Design review of the part built by this model. Coordinates are the model's own, in mm. Coordinates: 2 decimals unless noted, no trailing zeros. Order: outer loops, then holes, each group sorted by start corner. A loop starts at its lowest first (then second) coordinate and runs counter-clockwise, first axis right, second up. Notation, with made-up numbers: (27, 87) -> (43, 87) arc R27 cw to (43, 104) -> close; hole circle Ø8 at (-1, 31). An arc over 180 degrees is marked (long way). Use a Markdown table: item, result. Add a question column.
Q1. Add section B-B (y = -10). State the section outline as (x, z) points.
Q2. Add section A-A (x = 40). State the section outline as (y, z) points.
Q3. Wall thickness on probe 1 along Y at (x, z) = (40, 2.45); probe 2 along Y at (x, z) = (-37.1, 2.35); probe 3 along Y at (x, z) = (-20, 0.8): over which ranges is each line inside the solid? List them lowest first.
Q4. Add section D-D (x = -20). State the section outline as (y, z) points.
Q5. Add section C-C (y = 38). State the section outline as (x, z) points.
Q6. The part is to be moulded in two halves that separate along Y. For faces 1 (the face through (-50, -1, 1)), 2 (the face through (-34.79, -0.96, 1.52)), 3 (the face through (1, -44, 1)), 4 (the face through (-48.98, 43.04, 1.52)), say which applies: pulls with the +Y half, pulls with the -Y half, needs draft (parallel to the pull), parting line crosses it, or undercut.
Autodesk Inventor part; units mm, degrees
ref_plane "YZ Plane" through (0, 0, 0) normal (1, 0, 0) x (0, 1, 0)
ref_plane "XZ Plane" through (0, 0, 0) normal (0, 1, 0) x (-1, 0, 0)
ref_plane "XY Plane" through (0, 0, 0) normal (0, 0, 1) x (1, 0, 0)
sketch "Sketch1" plane through (0, 0, 0) normal (0, 0, 1) x (1, 0, 0)
  line L0 (-50, 44) -> (50, 44)
  line L1 (50, 44) -> (50, -44)
  line L2 (50, -44) -> (-50, -44)
  line L3 (-50, -44) -> (-50, 44)
  line L4 (0, 44) -> (0, -44) construction
  line L5 (-50, 0) -> (50, 0) construction
  point P0 (0, 0)
  dimension "d0" = 100
  dimension "d1" = 88
extrude "Extrusion1" add sketch "Sketch1" along normal blind 3
sketch "Sketch2" plane through (0, 0, 3) normal (0, 0, 1) x (1, 0, 0)
  line L0 (-50, 44) -> (-50, -44)
  line L1 (50, -44) -> (50, 44)
  circle A0 centre (0, 0) radius 2.5
  circle A1 centre (0, 10) radius 2.5
  line L2 (0, 0) -> (0, 20.5611) construction
  circle A2 centre (-10, 0) radius 2.5
  circle A3 centre (0, -10) radius 2.5
  circle A4 centre (10, 0) radius 2.5
  circle A5 centre (-37.1, 0) radius 2.5
  circle A6 centre (-37.1, -10) radius 2.5
  circle A7 centre (-37.1, -20) radius 2.5
  circle A8 centre (-37.1, 10) radius 2.5
  circle A9 centre (-37.1, 0) radius 2.5
  circle A10 centre (-37.1, -10) radius 2.5
  circle A11 centre (-37.1, 20) radius 2.5
  circle A12 centre (-37.1, 10) radius 2.5
  circle A13 centre (-37.1, 0) radius 2.5
  line L3 (0, 0) -> (-50, 0) construction
  circle A14 centre (40, 0) radius 3.6 construction
  circle A15 centre (40, 20) radius 3.6 construction
  circle A16 centre (40, -20) radius 3.6 construction
  circle A17 centre (40, 0) radius 3.6 construction
  circle A18 centre (40, 0) radius 3.6
  line L4 (40, 0) -> (40, 20) construction
  line L5 (40, 0) -> (40, -20) construction
  circle A19 centre (40, 20) radius 2.5
  circle A20 centre (40, -20) radius 2.5
  dimension "d40" = 6.5
  dimension "d4" = 5
  dimension "d5" = 5
  dimension "d6" = 10
  dimension "d9" = 360
  dimension "d11" = 5
  dimension "d12" = 12.9
  dimension "d15" = 10
  dimension "d18" = 10
  dimension "d28" = 20
  dimension "d31" = 20
  dimension "d64" = 7.2
  dimension "d65" = 5
  dimension "d66" = 5
extrude "Extrusion2" cut sketch "Sketch2" against normal up to next
sketch "Sketch3" plane through (0, 0, 3) normal (0, 0, 1) x (1, 0, 0)
  circle A0 centre (0, 0) radius 2.5
  line L0 (50, 44) -> (-50, 44)
  line L1 (-50, -44) -> (50, -44)
  line L2 (0, 0) -> (0, -39.6664) construction
  line L3 (0, 0) -> (-44.4767, 0) construction
  line L4 (-3.25, -38) -> (3.25, -38) construction
  line L5 (-3.25, -39.5) -> (3.25, -39.5)
  line L6 (3.25, -36.5) -> (-3.25, -36.5)
  arc A1 (-3.25, -36.5) -> (-3.25, -39.5) centre (-3.25, -38) ccw
  arc A2 (3.25, -39.5) -> (3.25, -36.5) centre (3.25, -38) ccw
  line L7 (16.9, -38) -> (23.4, -38) construction
  line L8 (16.9, -39.5) -> (23.4, -39.5)
  line L9 (23.4, -36.5) -> (16.9, -36.5)
  arc A3 (16.9, -36.5) -> (16.9, -39.5) centre (16.9, -38) ccw
  arc A4 (23.4, -39.5) -> (23.4, -36.5) centre (23.4, -38) ccw
  line L10 (-23.4, -38) -> (-16.9, -38) construction
  line L11 (-23.4, -39.5) -> (-16.9, -39.5)
  line L12 (-16.9, -36.5) -> (-23.4, -36.5)
  arc A5 (-23.4, -36.5) -> (-23.4, -39.5) centre (-23.4, -38) ccw
  arc A6 (-16.9, -39.5) -> (-16.9, -36.5) centre (-16.9, -38) ccw
  line L13 (-3.25, -38) -> (3.25, -38) construction
  line L14 (-3.25, -39.5) -> (3.25, -39.5)
  line L15 (3.25, -36.5) -> (-3.25, -36.5)
  arc A7 (-3.25, -36.5) -> (-3.25, -39.5) centre (-3.25, -38) ccw
  arc A8 (3.25, -39.5) -> (3.25, -36.5) centre (3.25, -38) ccw
  line L16 (-3.25, 38) -> (3.25, 38) construction
  line L17 (-3.25, 39.5) -> (3.25, 39.5)
  line L18 (3.25, 36.5) -> (-3.25, 36.5)
  arc A9 (-3.25, 39.5) -> (-3.25, 36.5) centre (-3.25, 38) ccw
  arc A10 (3.25, 36.5) -> (3.25, 39.5) centre (3.25, 38) ccw
  arc A11 (16.9, 39.5) -> (16.9, 36.5) centre (16.9, 38) ccw
  line L19 (23.4, 36.5) -> (16.9, 36.5)
  line L20 (16.9, 38) -> (23.4, 38) construction
  line L21 (16.9, 39.5) -> (23.4, 39.5)
  arc A12 (23.4, 36.5) -> (23.4, 39.5) centre (23.4, 38) ccw
  arc A13 (-23.4, 39.5) -> (-23.4, 36.5) centre (-23.4, 38) ccw
  line L22 (-16.9, 36.5) -> (-23.4, 36.5)
  line L23 (-23.4, 38) -> (-16.9, 38) construction
  line L24 (-23.4, 39.5) -> (-16.9, 39.5)
  arc A14 (-16.9, 36.5) -> (-16.9, 39.5) centre (-16.9, 38) ccw
  arc A15 (-3.25, 39.5) -> (-3.25, 36.5) centre (-3.25, 38) ccw
  line L25 (3.25, 36.5) -> (-3.25, 36.5)
  line L26 (-3.25, 38) -> (3.25, 38) construction
  line L27 (-3.25, 39.5) -> (3.25, 39.5)
  arc A16 (3.25, 36.5) -> (3.25, 39.5) centre (3.25, 38) ccw
  line L28 (50, -44) -> (-50, -44)
  line L29 (0, -44) -> (0, -31) construction
  line L30 (-10.32, -31) -> (10.32, -31) construction
  line L31 (-10.32, -33.5) -> (10.32, -33.5)
  line L32 (10.32, -28.5) -> (-10.32, -28.5)
  arc A17 (-10.32, -28.5) -> (-10.32, -33.5) centre (-10.32, -31) ccw
  arc A18 (10.32, -33.5) -> (10.32, -28.5) centre (10.32, -31) ccw
  line L33 (-10.32, 33.5) -> (10.32, 33.5)
  line L34 (10.32, 28.5) -> (-10.32, 28.5)
  arc A19 (-10.32, 33.5) -> (-10.32, 28.5) centre (-10.32, 31) ccw
  line L35 (0, 44) -> (0, 31) construction
  line L36 (-10.32, 31) -> (10.32, 31) construction
  line L37 (-10.32, 33.5) -> (10.32, 33.5)
  line L38 (10.32, 28.5) -> (-10.32, 28.5)
  arc A20 (-10.32, 33.5) -> (-10.32, 28.5) centre (-10.32, 31) ccw
  arc A21 (10.32, 28.5) -> (10.32, 33.5) centre (10.32, 31) ccw
  point P0 (0, -38)
  point P1 (20.15, -38)
  point P2 (-20.15, -38)
  point P3 (0, -38)
  point P4 (0, 38)
  point P5 (20.15, 38)
  point P6 (-20.15, 38)
  point P7 (0, 38)
  dimension "d38" = 3
  dimension "d40" = 6.5
  dimension "d43" = 20.15
  dimension "d46" = 20.15
  dimension "d59" = 6
  dimension "d61" = 13
  dimension "d62" = 10.32
  dimension "d63" = 5
extrude "Extrusion3" cut sketch "Sketch3" against normal up to next contours A1 L6 A2 L5 | A3 L9 A4 L8 | A5 L12 A6 L11 | L17 A10 L18 A9 | L21 A12 L19 A11 | L24 A14 L22 A13 | A17 L32 A18 L31 | L33 A21 L34 A19
fillet "Fillet1" radius 3.38 4 edges at (50, -44, 1.5) (50, 44, 1.5) (-50, -44, 1.5) (-50, 44, 1.5)
sketch "Sketch5" plane through (0, 0, 3) normal (0, 0, 1) x (1, 0, 0)
  line L0 (-20, 20) -> (20, 20) construction
  line L1 (20, 20) -> (20, -20) construction
  line L2 (20, -20) -> (-20, -20) construction
  line L3 (-20, -20) -> (-20, 20) construction
  circle A0 centre (0, 0) radius 2.5
  line L4 (-20, 20) -> (20, -20) construction
  line L5 (20, 20) -> (-20, -20) construction
  circle A1 centre (-20, 20) radius 2.75
  circle A2 centre (20, 20) radius 2.75
  circle A3 centre (-20, -20) radius 2.75
  circle A4 centre (20, -20) radius 2.75
  dimension "d67" = 40
  dimension "d68" = 40
  dimension "d69" = 5.5
  dimension "d70" = 5.5
  dimension "d71" = 5.5
  dimension "d72" = 5.5
extrude "Extrusion5" cut sketch "Sketch5" against normal through all contours A1 | A2 | A3 | A4
properties part number "20mm gantry plate" material "Aluminum 6061"
Established:
| question | item | result |
|---|---|---|
| 1 | outline | (-50, 0) -> (-39.6, 0) -> (-39.6, 3) -> (-50, 3) -> close; (-34.6, 0) -> (-2.5, 0) -> (-2.5, 3) -> (-34.6, 3) -> close; (2.5, 0) -> (50, 0) -> (50, 3) -> (2.5, 3) -> close |
| 2 | outline | (-44, 0) -> (-22.5, 0) -> (-22.5, 3) -> (-44, 3) -> close; (-17.5, 0) -> (-3.6, 0) -> (-3.6, 3) -> (-17.5, 3) -> close; (3.6, 0) -> (17.5, 0) -> (17.5, 3) -> (3.6, 3) -> close; (22.5, 0) -> (44, 0) -> (44, 3) -> (22.5, 3) -> close |
| 3 | probe 1 | -44 to -22.5, -17.5 to -3.6, 3.6 to 17.5, 22.5 to 44 |
| 3 | probe 2 | -44 to -22.5, -17.5 to -12.5, -7.5 to -2.5, 2.5 to 7.5, 12.5 to 17.5, 22.5 to 44 |
| 3 | probe 3 | -44 to -39.5, -36.5 to -22.75, -17.25 to 17.25, 22.75 to 36.5, 39.5 to 44 |
| 4 | outline | (-44, 0) -> (-39.5, 0) -> (-39.5, 3) -> (-44, 3) -> close; (-36.5, 0) -> (-22.75, 0) -> (-22.75, 3) -> (-36.5, 3) -> close; (-17.25, 0) -> (17.25, 0) -> (17.25, 3) -> (-17.25, 3) -> close; (22.75, 0) -> (36.5, 0) -> (36.5, 3) -> (22.75, 3) -> close; (39.5, 0) -> (44, 0) -> (44, 3) -> (39.5, 3) -> close |
| 5 | outline | (-50, 0) -> (-24.9, 0) -> (-24.9, 3) -> (-50, 3) -> close; (-15.4, 0) -> (-4.75, 0) -> (-4.75, 3) -> (-15.4, 3) -> close; (4.75, 0) -> (15.4, 0) -> (15.4, 3) -> (4.75, 3) -> close; (24.9, 0) -> (50, 0) -> (50, 3) -> (24.9, 3) -> close |
| 6 | face 1 | needs draft |
| 6 | face 2 | undercut |
| 6 | face 3 | pulls with the -Y half |
| 6 | face 4 | pulls with the +Y half |
